from build123d import *

# Parameters (mm, degrees)
SKETCH1_R           = 4.95
BOSS_EXTRUDE2_DEPTH = 7


with BuildPart() as part:
    # Sketch1 → Boss-Extrude2 (new body)
    with BuildSketch(Plane(origin=(0, 0, 0), x_dir=(1, 0, 0), z_dir=(0, 1, 0))):
        with BuildLine():
            ThreePointArc((-8, 7.716425662), (-11.115, 0), (-8, -7.716425662))
            Line((-8, -7.716425662), (8, -7.716425662))
            ThreePointArc((8, -7.716425662), (11.115, 0), (8, 7.716425662))
            Line((8, 7.716425662), (-8, 7.716425662))
        make_face()
        with Locations(Location((0, 0, 0), (0, 0, 270))):
            Circle(SKETCH1_R, mode=Mode.SUBTRACT)
    extrude(amount=BOSS_EXTRUDE2_DEPTH)


solid = part.part
The listing builds one solid part. Answer for the finished solid, in the listing's coordinates (mm). Give positions to 0.01 mm unless a question says otherwise; leave off trailing zeros. Write each loop counter-clockwise with the first axis right and the second up, starting at its lowest first coordinate (ties: lowest second). Pieces come first, ordered by that corner, then holes. Notation, with made-up numbers: (1, 57.25) -> (46, 57.25) arc R23 cw to (46, 95.25) -> close; hole circle Ø1 at (66.25, 10.5). An arc over 180 degrees is marked (long way). One line per question, with ' | ' between items. Start each with the question number.
1. Section A-A (z = 0) is taken. Determine the outline of the cut face in (x, y) (3 decimals).
2. Section C-C (x = 0) is taken. Determine the outline of the cut face in (y, z), plus the area to 3 significant figures.
3. Section B-B (y = 4) is taken. Determine the outline of the cut face in (x, z) (3 decimals), plus the area to 3 significant figures.
4. Find the intervals of material crossed by probe 1 along X at (y, z) = (0.75, 1); probe 2 along X at (y, z) = (6, -1.75); probe 3 along Z at (x, y) = (0.75, 0.75), in increasing order.
5. Section D-D (x = -9) is taken. Determine the outline of the cut face in (y, z), plus the area to 3 significant figures.
6. Given pin 1 Ø1 at (y, z) = (1.5, -2.5) entering from -X, flat-ended and moving along its own axis, determine where the tip first touches the part or whether it passes through.
7. For a pull along Z with two mould halves and no side action, classify faces 1 (the cylindrical face through (-11.114, 3.451, -0.119)), 2 (the cylindrical face through (1.49, 3.45, 4.72)), 3 (the flat face through (0, 3, 7.716)) as pulls with the +Z half, pulls with the -Z half, needs draft (parallel to the pull), parting line crosses it, or undercut.
Response values:
1) outline: (-11.115, 0) -> (-4.95, 0) -> (-4.95, 7) -> (-11.115, 7) -> close; (4.95, 0) -> (11.115, 0) -> (11.115, 7) -> (4.95, 7) -> close
2) outline: (0, -7.72) -> (7, -7.72) -> (7, -4.95) -> (0, -4.95) -> close; (0, 4.95) -> (7, 4.95) -> (7, 7.72) -> (0, 7.72) -> close | area: 38.7 mm2
3) outline: (-8, -7.716) -> (8, -7.716) arc R11.115 ccw to (8, 7.716) -> (-8, 7.716) arc R11.115 ccw to start; hole circle Ø9.9 at (0, 0) | area: 236 mm2
4) probe 1: -11.07 to -4.85, 4.85 to 11.07 | probe 2: -10.98 to -4.63, 4.63 to 10.98 | probe 3: -7.72 to -4.89, 4.89 to 7.72
5) outline: (0, -6.52) -> (7, -6.52) -> (7, 6.52) -> (0, 6.52) -> close | area: 91.3 mm2
6) pin 1: x = -10.93
7) face 1: parting line crosses it | face 2: undercut | face 3: pulls with the +Z half
